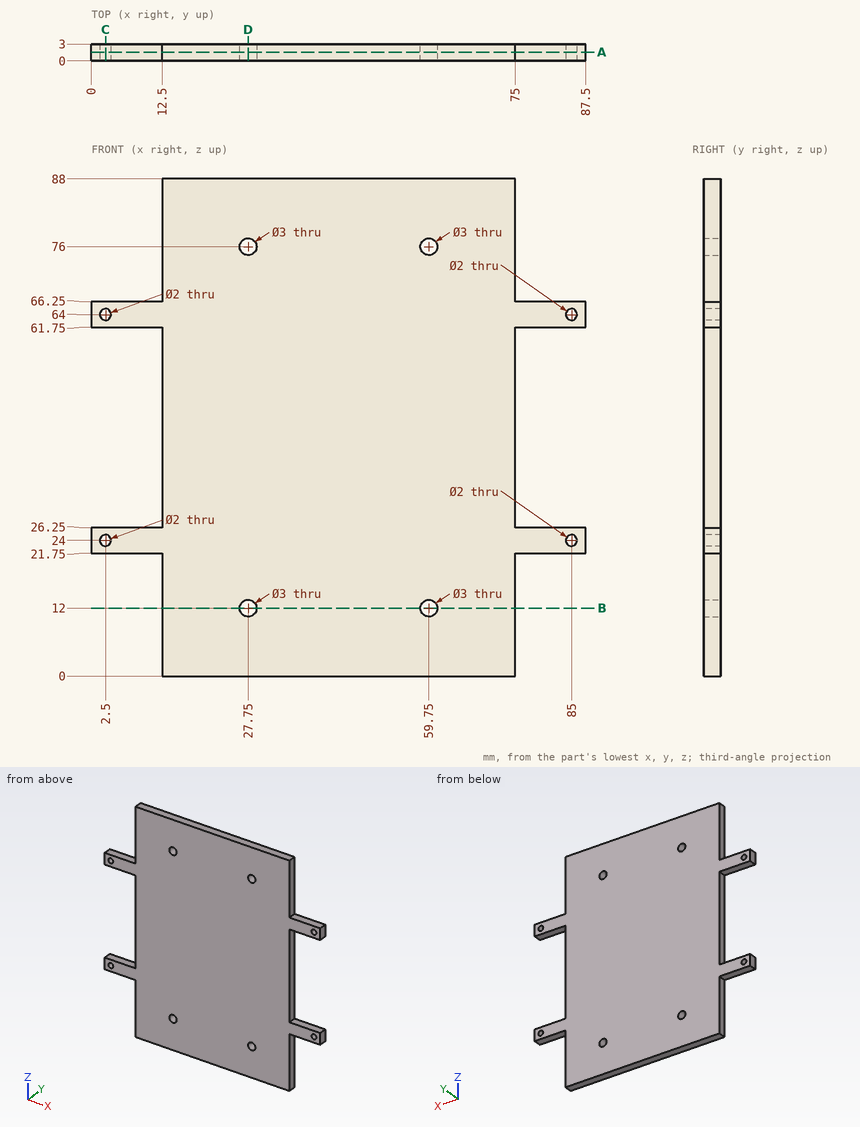
Answer from the drawing. Dimensions are ordinates in mm from the lowest x, y and z of the part. Give positions to 0.01 mm unless a question says otherwise; leave off trailing zeros. Loops run counter-clockwise (first coordinate to the right, second up) from the corner with the lowest first, then second, coordinate; pieces in that order, holes last. Notation, with made-up numbers: (17, 16.5) - (44, 16.5) arc R25 cw to (44, 47.5) - close; hole circle Ø11 at (56.25, 20). An arc over 180 degrees is marked (long way). Answer as a JSON object with one key per item and string values.
1. A cutting plane is placed at C-C (x = 2.5). Write down the section's boundary in (y, z).
Determined:
{"outline": "(0, 21.75) - (3, 21.75) - (3, 23) - (0, 23) - close; (0, 25) - (3, 25) - (3, 26.25) - (0, 26.25) - close; (0, 61.75) - (3, 61.75) - (3, 63) - (0, 63) - close; (0, 65) - (3, 65) - (3, 66.25) - (0, 66.25) - close"}
2. A cutting plane is placed at A-A (y = 1.55). Give the number of separate pieces and of enclosed holes in the cut face, then the cut area to 3 significant figures.
Determined:
{"separate pieces": "1", "enclosed holes": "8", "area": "5,680 mm²"}
3. A cutting plane is placed at D-D (x = 27.75). Write down the section's boundary in (y, z), then the cut area to 3 significant figures.
Determined:
{"outline": "(0, 0) - (3, 0) - (3, 10.5) - (0, 10.5) - close; (0, 13.5) - (3, 13.5) - (3, 74.5) - (0, 74.5) - close; (0, 77.5) - (3, 77.5) - (3, 88) - (0, 88) - close", "area": "246 mm²"}
4. A cutting plane is placed at B-B (z = 12). Write down the section's boundary in (x, y), then the cut area to 4 significant figures.
Determined:
{"outline": "(12.5, 0) - (26.25, 0) - (26.25, 3) - (12.5, 3) - close; (29.25, 0) - (58.25, 0) - (58.25, 3) - (29.25, 3) - close; (61.25, 0) - (75, 0) - (75, 3) - (61.25, 3) - close", "area": "169.5 mm²"}
5. Flat-ended cylindrical pins translate along their axes: pin 1 Ø1.5 at (y, z) = (1, 51) entering from +X; pin 2 Ø1.5 at (x, y) = (80, 1.5) entering from -Z. Find the tip coordinate at first contact, or state that the pin passes through.
Determined:
{"pin 1": "x = 75", "pin 2": "z = 21.75"}
6. Find the intervals of material crossed by L1, parallel to Z at x = 2.5, y = 2.2; L2, parallel to Z at x = 27.75, y = 1.7; L3, parallel to X at y = 1.7, z = 76, in increasing order. Write a range as [from, to].
Determined:
{"L1": "[21.75, 23], [25, 26.25], [61.75, 63], [65, 66.25]", "L2": "[0, 10.5], [13.5, 74.5], [77.5, 88]", "L3": "[12.5, 26.25], [29.25, 58.25], [61.25, 75]"}
